Check sheet for the modelled part. Datum: model origin and axes. Units: mm. A direction names the side the tool comes from. Give positions to 0.01 mm unless a question says otherwise; leave off trailing zeros. Write each loop counter-clockwise with the first axis right and the second up, starting at its lowest first coordinate (ties: lowest second). Pieces come first, ordered by that corner, then holes. Notation, with made-up numbers: M 74.5,20.25 L 118.5,20.25 A24 ccw 118.5,42.25 Z; hole C -2.5,67.5 d5. An arc over 180 degrees is marked long. Use CSV: the item, a comma, the result in double quotes. Start each with the question number.
1. Cross-section at C-C, the plane y = -8. Enter the section's corners in (x, z).
2. Mould release check, pull along Z, two halves, no side actions. Record for faces 1 (the face through (14, 0, 1)), 2 (the face through (-4, 0, 6.5)), 3 (the face through (-10, 0, 3)): +Z half, -Z half, draft (parallel to the pull), parting line (faces both ways), or undercut.
3. Access from +Z, -Z, +X, -X, +Y, -Y to the whole of each face (thin tool, end or side, straight path). Record for faces 4 (the face through (-3, 0, 5.5)), 5 (the face through (14, 0, 11)).
4. Cross-section at B-B, the plane z = 1. Enter the section's corners in (x, y), and give its area (3 significant figures).
5. Depth check by flat-ended pin: P1, Ø3, axis at y = 4.5, z = 6.5, coming from the -X side; P2, Ø2, axis at x = -6.5, z = 8, coming from the +Y side; P3, Ø1, axis at y = -6.5, z = 2.5, coming from the -X side. Enter the tip coordinate at first touch or a pass-through.
6. Cross-section at A-A, the plane x = 7.75. Enter the section's corners in (y, z) (3 decimals), and give its area (3 significant figures).
7. Scan lines: line 1 (Z direction, x = -0.25, y = 5.5); line 2 (X direction, y = 2.5, z = 6.25); line 3 (X direction, y = -0.5, z = 4.75). Record each from-to range of solid material in increasing order.
8. Cross-section at D-D, the plane x = -1.5. Enter the section's corners in (y, z), and give its area (3 significant figures).
from build123d import *

# Parameters (mm, degrees)
F1_DEPTH = 12
F3_DEPTH = 20.001
F4_SIZE  = 2
F2_W     = 10
F2_H     = 1
F9_DEPTH = 25


with BuildPart() as f1:
    # F0 (on Top) → F1 (new body)
    with BuildSketch(Plane.XY):
        with BuildLine():
            Line((15, 10), (0, 10))
            Line((0, 10), (0, 2.75))
            ThreePointArc((0, 2.75), (1.9445436483, 1.9445436483), (2.75, 0))
            ThreePointArc((2.75, 0), (1.9445436483, -1.9445436483), (0, -2.75))
            Line((0, -2.75), (0, -10))
            Line((0, -10), (15, -10))
            Line((15, -10), (15, 10))
        make_face()
        with BuildLine():
            Line((0, 2.75), (0, 10))
            ThreePointArc((0, 10), (-10, 0), (0, -10))
            Line((0, -10), (0, -2.75))
            ThreePointArc((0, -2.75), (-2.75, 0), (0, 2.75))
        make_face()
    extrude(amount=F1_DEPTH)

    # F2 (on face) → F3 (cut, through all)
    with BuildSketch(Plane.XZ.offset(10)):
        with BuildLine():
            Line((7.75, 6.5), (7.75, 5.5))
            Line((7.75, 5.5), (3.529514246, 5.5))
            ThreePointArc((3.529514246, 5.5), (8.0004351666, 1.7573849777), (12, 6))
            ThreePointArc((12, 6), (8.0004351666, 10.2426150223), (3.529514246, 6.5))
            Line((3.529514246, 6.5), (7.75, 6.5))
        make_face()
        with BuildLine():
            Line((3.529514246, 5.5), (7.75, 5.5))
            Line((7.75, 5.5), (7.75, 6.5))
            Line((7.75, 6.5), (3.529514246, 6.5))
            ThreePointArc((3.529514246, 6.5), (3.5, 6), (3.529514246, 5.5))
        make_face()
    extrude(amount=-F3_DEPTH, mode=Mode.SUBTRACT)

    # F4
    f4_edges = [f1.edges().sort_by_distance(p)[0] for p in [
        (15, 0, 0),
        (15, 0, 12),
    ]]
    chamfer(f4_edges, length=F4_SIZE)

    # F8: sweep along a path in F7
    with BuildLine(Plane.XZ) as f8_path:
        CenterArc((7.75, 6), 4.25, 0, 360)
    # F6 (on mid) → F8 (sweep)
    with BuildSketch(Plane.XY.offset(6)):
        with BuildLine():
            Line((3.5, 2.5), (3.5, -2.5))
            ThreePointArc((3.5, -2.5), (4.5, 0), (3.5, 2.5))
        make_face()
    sweep(path=f8_path.line)

    # F2 (on face) → F9 (cut)
    with BuildSketch(Plane.XZ.offset(10)):
        with BuildLine():
            Line((3.529514246, 5.5), (7.75, 5.5))
            Line((7.75, 5.5), (7.75, 6.5))
            Line((7.75, 6.5), (3.529514246, 6.5))
            ThreePointArc((3.529514246, 6.5), (3.5, 6), (3.529514246, 5.5))
        make_face()
        with BuildLine():
            Line((0, 5.5), (3.529514246, 5.5))
            ThreePointArc((3.529514246, 5.5), (3.5, 6), (3.529514246, 6.5))
            Line((3.529514246, 6.5), (0, 6.5))
            Line((0, 6.5), (0, 5.5))
        make_face()
        with Locations((-5, 6)):
            Rectangle(F2_W, F2_H)
    extrude(amount=-F9_DEPTH, mode=Mode.SUBTRACT)


solid = f1.part
Worked answers:
1,outline,"M -6,0 L 13,0 L 15,2 L 15,10 L 13,12 L -6,12 L -6,6.5 L 3.53,6.5 A4.25 cw long 3.53,5.5 L -6,5.5 Z"
2,face 1,"-Z half"
2,face 2,"undercut"
2,face 3,"draft"
3,face 4,"-X, +Y, -Y"
3,face 5,"+Z, +X, +Y, -Y"
4,outline,"M 0,-10 L 14,-10 L 14,10 L 0,10 A10 ccw Z; hole C 0,0 d5.5"
4,area,"413 mm^2"
5,P1,"stops at x = -9.54"
5,P2,"stops at y = 8.35"
5,P3,"stops at x = -8"
6,outline,"M -10,0 L 10,0 L 10,1.75 L 2.5,1.75 A3.625 ccw -2.5,1.75 L -10,1.75 Z; M -10,10.25 L -2.5,10.25 A3.625 ccw 2.5,10.25 L 10,10.25 L 10,12 L -10,12 Z"
6,area,"76.9 mm^2"
7,line 1,"z = 0 to 5.5, 6.5 to 12"
7,line 2,"x = 11.99 to 15"
7,line 3,"x = -9.99 to -2.7, 2.7 to 4.71, 10.79 to 15"
8,outline,"M -9.89,0 L -2.3,0 L -2.3,5.5 L -9.89,5.5 Z; M -9.89,6.5 L -2.3,6.5 L -2.3,12 L -9.89,12 Z; M 2.3,0 L 9.89,0 L 9.89,5.5 L 2.3,5.5 Z; M 2.3,6.5 L 9.89,6.5 L 9.89,12 L 2.3,12 Z"
8,area,"167 mm^2"
